Read the model definition and answer for the solid it produces. Units are mm, in the model's axes. A direction names the side the tool comes from. Give positions to 0.01 mm unless a question says otherwise; leave off trailing zeros. Write each loop counter-clockwise with the first axis right and the second up, starting at its lowest first coordinate (ties: lowest second). Pieces come first, ordered by that corner, then holes. Notation, with made-up numbers: M 0,-1.5 L 43,-1.5 A18 cw 43,28.5 Z; hole C -14.5,-39.5 d9. An arc over 180 degrees is marked long. Use a Markdown table: item, result. Add a question column.
Item 1: For faces 1 (the flat face through (0.81, 2.14, 1.37)), 2 (the conical face through (-2.575, 0.33, 0.811)), determine the directions among +Z, -Z, +X, -X, +Y, -Y from which every point of the face is accessible in a straight line to the end or side of a thin tool.
Item 2: A cutting plane is placed at B-B on y = -12. Determine the outline of the cut face in (x, z), then the cut area to 3 significant figures.
Item 3: The mould has two halves that part along Z. Classify faces 3 (the cylindrical face through (1.3, -9.71, -2.03)), 4 (the flat face through (0.961, 0.616, -0.013)), 5 (the flat face through (-2, 3.23, 0)): pulls with the +Z half, pulls with the -Z half, needs draft (parallel to the pull), parting line crosses it, or undercut.
Item 4: Given P1, Ø1, axis at y = -8.5, z = 2.5, coming from the -X side; P2, Ø1, axis at x = -4, z = -2.5, coming from the -Y side; P3, Ø5, axis at y = -2, z = 0.5, coming from the +X side, each flat-ended and moving along its own axis, determine where each tip first touches the part or whether it passes through.
Item 5: A cutting plane is placed at A-A on y = 1.5. Determine the outline of the cut face in (x, z).
Item 6: Consider probe 1 along Y at (x, z) = (-1, 4.5); probe 2 along X at (y, z) = (-4.25, 0.75); probe 3 along Y at (x, z) = (3, 0.5). Determine where each line is inside the solid, lowest interval first. Write a range as [from, to].
Autodesk Inventor part; units mm, degrees
ref_plane "YZ Plane" through (0, 0, 0) normal (1, 0, 0) x (0, 1, 0)
ref_plane "XZ Plane" through (0, 0, 0) normal (0, 1, 0) x (-1, 0, 0)
ref_plane "XY Plane" through (0, 0, 0) normal (0, 0, 1) x (1, 0, 0)
sketch "Sketch1" plane through (0, 0, 0) normal (0, 0, 1) x (1, 0, 0)
  line L0 (0, 0) -> (0, 3.23)
  line L1 (0, 3.23) -> (-5.22, 3.23)
  line L2 (-5.22, 3.23) -> (-5.22, 7.9668) construction
  line L3 (-2.4122, 0) -> (-5.22, 3.23)
  line L4 (0, 0) -> (-2.4122, 0)
  line L5 (-5.22, 3.23) -> (-8.3852, 6.8711) construction
  line L6 (-4.6965, 2.6278) -> (0, 2.6278) construction
  dimension "d0" = 3.23
  dimension "d3" = 41
  dimension "d23" = 5.22
  dimension "d25" = 4.6965
revolve "Revolution1" add sketch "Sketch1" angle 360 about axis through (0, 0, 0) along (0, 1, 0)
sketch "Sketch2" plane through (0, 0, 0) normal (0, -1, 0) x (1, 0, 0)
  circle A0 centre (0, 0) radius 2.4122
  dimension "d22" = 4.8244
extrude "Extrusion1" add sketch "Sketch2" along normal blind 20
sketch "Sketch3" plane through (0, 3.23, 0) normal (0, 1, 0) x (1, 0, 0)
  line L0 (0, -1.836) -> (-1.59, -0.918)
  line L1 (-1.59, -0.918) -> (-1.59, 0.918)
  line L2 (-1.59, 0.918) -> (0, 1.836)
  line L3 (0, 1.836) -> (1.59, 0.918)
  line L4 (1.59, 0.918) -> (1.59, -0.918)
  line L5 (1.59, -0.918) -> (0, -1.836)
  point P0 (0, 0)
  point P1 (0, 0)
  dimension "d8" = 3.18
extrude "Extrusion2" cut sketch "Sketch3" against normal blind 2.21
sketch "Sketch4" plane through (0, 0, 0) normal (0, 0, 1) x (1, 0, 0)
  line L0 (1.59, 1.02) -> (0, 0)
sketch "Sketch5" plane through (0, 1.02, 0) normal (0, 1, 0) x (1, 0, 0)
  line L0 (0, -1.836) -> (-1.59, -0.918)
  line L1 (1.59, -0.918) -> (0, -1.836)
  line L2 (1.59, 0.918) -> (1.59, -0.918)
  line L3 (0, 1.836) -> (1.59, 0.918)
  line L4 (-1.59, 0.918) -> (0, 1.836)
  line L5 (-1.59, -0.918) -> (-1.59, 0.918)
  point P0 (0, 0)
sketch "Sketch6" plane through (0, 0, 0) normal (0, 1, 0) x (-1, 0, 0)
  point P0 (0, 0)
  point P1 (0, 0)
sketch "Sketch7" plane through (0, 0, 0) normal (1, 0, 0) x (0, 1, 0)
  line L0 (1.02, -1.836) -> (0, 0)
loft "Loft1" cut section 1 edges at (-0.795, 1.02, 1.377) (0.795, 1.02, 1.377) (1.59, 1.02, 0) (0.795, 1.02, -1.377) (-0.795, 1.02, -1.377) (-1.59, 1.02, 0) section 2 point at (0, 0, 0)
chamfer "Chamfer1" distance 0.5 angle 45 1 edges at (-2.4122, -20, 0)
thread "Thread1"
fillet "Fillet1" radius 0.5 2 edges at (0, 0, -2.4122) (0, 0, 2.4122)
fillet "Fillet2" radius 0.04 1 edges at (5.22, 3.23, 0)
properties part number "CountersunkBolt" material "Steel, Carbon"
Filled in:
| question | item | result |
|---|---|---|
| 1 | face 1 | +Y |
| 1 | face 2 | -Y |
| 2 | outline | C 0,0 d4.82 |
| 2 | area | 18.3 mm² |
| 3 | face 3 | parting line crosses it |
| 3 | face 4 | undercut |
| 3 | face 5 | needs draft |
| 4 | P1 | x = -1.35 |
| 4 | P2 | y = 2.08 |
| 4 | P3 | x = 2.82 |
| 5 | outline | C 0,0 d7.43; hole M -1.59,-0.92 L 0,-1.84 L 1.59,-0.92 L 1.59,0.92 L 0,1.84 L -1.59,0.92 Z |
| 6 | probe 1 | [2.53, 3.23] |
| 6 | probe 2 | [-2.29, 2.29] |
| 6 | probe 3 | [0.72, 3.23] |
